Part model, mm, in its own coordinate system. A direction names the side the tool comes from. Give positions to 0.01 mm unless a question says otherwise; leave off trailing zeros. Order: outer loops, then holes, each group sorted by start corner. A loop starts at its lowest first (then second) coordinate and runs counter-clockwise, first axis right, second up. Notation, with made-up numbers: (77.5, 42.5) - (105.5, 42.5) arc R22 cw to (105.5, 78.5) - close; hole circle Ø9 at (4.5, -18). An arc over 180 degrees is marked (long way). One line per item, written item: value.
```python
from build123d import *

# Parameters (mm, degrees)
BASEHEAD_DEPTH = 4
BODYSKE_W      = 94
BODYSKE_H      = 3


with BuildPart() as part:
    # Sketch1 → BaseHead (new body)
    with BuildSketch(Plane(origin=(0, 0, 0), x_dir=(0, 0, -1), z_dir=(1, 0, 0))):
        Polygon((5, 2.886751346), (5, -2.886751346), (0, -5.773502692), (-5, -2.886751346), (-5, 2.886751346), (0, 5.773502692), align=None)
    extrude(amount=BASEHEAD_DEPTH)

    # BodySke → BaseBody (revolve)
    with BuildSketch(Plane.XY):
        with Locations((47, 1.5)):
            Rectangle(BODYSKE_W, BODYSKE_H)
    revolve(axis=Axis((0, 0, 0), (1, 0, 0)))

    # Sketch3 → HeadChamfer (revolve, cut)
    with BuildSketch(Plane.XY):
        Polygon((0, 5), (3.333333333, 10.773502692), (3.333333333, 15.773502692), (-10, 15.773502692), (-10, 5), align=None)
    revolve(axis=Axis((0, 0, 0), (1, 0, 0)), mode=Mode.SUBTRACT)


solid = part.part
```
1) Slice it at A-A on x = 56. Write the cut outline in (y, z).
Answer:
outline: circle Ø6 at (0, 0)
2) Wall check: line 1 along X through (y, z) = (3.5, -1.5); line 2 along Y through (x, z) = (81.5, 0.25); line 3 along Y through (x, z) = (7, -2.25). Give the ranges that are in metal, low to high. Write a range as [from, to].
Answer:
line 1: x = [0, 4]
line 2: y = [-2.99, 2.99]
line 3: y = [-1.98, 1.98]
3) Drop flat-ended pins along their axis: P1, Ø2, axis at x = 80, z = -1.5, coming from the +Y side; P2, Ø2, axis at x = 80, z = 0, coming from the -Y side; P3, Ø3, axis at x = 84, y = -3.5, coming from the +Z side. Give the stop position or say it passes through.
Answer:
P1: stops at y = 2.96
P2: stops at y = -3
P3: stops at z = 2.24
4) Which spindle directions (+Z, -Z, +X, -X, +Y, -Y) get a long thin tool onto all of the face, cutting with end or side? Do faces 1 (the face through (4, -2.5, 2.2)), 2 (the face through (0.11, 2.6, 4.49)). Say none if no direction does.
Answer:
face 1: +X
face 2: +Z, -X, +Y
